from build123d import *

# Parameters (mm, degrees)
SKETCH1_W           = 34
SKETCH1_H           = 103
BOSS_EXTRUDE1_DEPTH = 0.5
SKETCH3_R           = 6.75
SKETCH3_W           = 7
SKETCH3_H           = 3.25
CUT_EXTRUDE1_DEPTH  = 55.242511004


with BuildPart() as part:
    # Sketch1 → Boss-Extrude1 (new, symmetric)
    with BuildSketch(Plane.XY):
        Rectangle(SKETCH1_W, SKETCH1_H)
    extrude(amount=BOSS_EXTRUDE1_DEPTH, both=True)

    # Sketch3 → Cut-Extrude1 (cut, through all)
    with BuildSketch(Plane.XY.offset(0.5)):
        with Locations((-0.255791225, 31.827660642)):
            Circle(SKETCH3_R)
        with Locations((-0.255791225, 10.237617462)):
            Circle(SKETCH3_R)
        with Locations((-0.255791225, -11.352425718)):
            Circle(SKETCH3_R)
        with Locations((-0.25, 45.125)):
            Rectangle(SKETCH3_W, SKETCH3_H)
    extrude(amount=-CUT_EXTRUDE1_DEPTH, mode=Mode.SUBTRACT)


solid = part.part
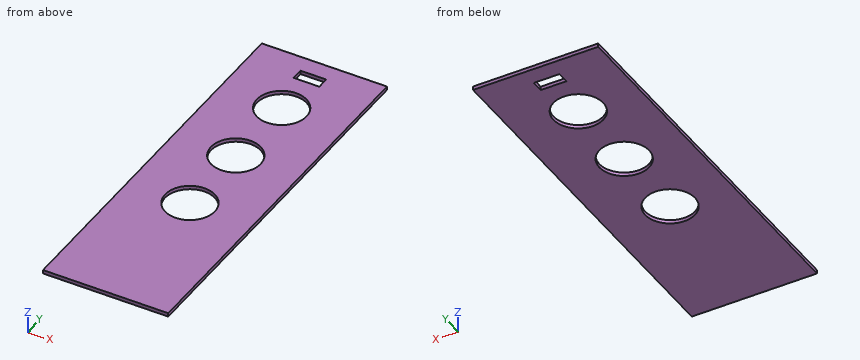
Part model, mm, in its own coordinate system. Round coordinates to 2 decimals unless told otherwise and drop trailing zeros. Write each loop counter-clockwise with the first axis right and the second up, starting at its lowest first coordinate (ties: lowest second). Pieces come first, ordered by that corner, then holes. Notation, with made-up numbers: (75, -20.5) - (108, -20.5) arc R22 cw to (108, 6.5) - close; hole circle Ø2 at (-12.75, 63.25). An arc over 180 degrees is marked (long way). Use CSV: the item, a comma, the result in double quotes.
Item 1: Wall check: L1, parallel to Y at x = 1, z = 0.4; L2, parallel to X at y = 45, z = 0.1; L3, parallel to X at y = -11, z = 0.05 (3 decimals). Give the ranges that are in metal, low to high.
Results list:
L1,"y = -51.5 to -17.98, -4.72 to 3.61, 16.87 to 25.2, 38.46 to 43.5, 46.75 to 51.5"
L2,"x = -17 to -3.75, 3.25 to 17"
L3,"x = -17 to -6.997, 6.485 to 17"
Item 2: Slice it at C-C, the plane y = 33. Write the cut outline in (x, z).
Results list:
outline,"(-17, -0.5) - (-6.9, -0.5) - (-6.9, 0.5) - (-17, 0.5) - close; (6.39, -0.5) - (17, -0.5) - (17, 0.5) - (6.39, 0.5) - close"
Item 3: Flat gauge pin, fed straight in: P1, Ø17.5, axis at x = -0.26, y = -11.35, coming from the -Z side. Where does the tip first touch, or does it go through?
Results list:
P1,"stops at z = -0.5"
Item 4: Slice it at A-A, the plane x = -1. Write the cut outline in (y, z), then the cut area to 3 significant figures.
Results list:
outline,"(-51.5, -0.5) - (-18.06, -0.5) - (-18.06, 0.5) - (-51.5, 0.5) - close; (-4.64, -0.5) - (3.53, -0.5) - (3.53, 0.5) - (-4.64, 0.5) - close; (16.95, -0.5) - (25.12, -0.5) - (25.12, 0.5) - (16.95, 0.5) - close; (38.54, -0.5) - (43.5, -0.5) - (43.5, 0.5) - (38.54, 0.5) - close; (46.75, -0.5) - (51.5, -0.5) - (51.5, 0.5) - (46.75, 0.5) - close"
area,"59.5 mm²"
Item 5: Slice it at D-D, the plane y = -6. Write the cut outline in (x, z), then the cut area to 3 significant figures.
Results list:
outline,"(-17, -0.5) - (-4.37, -0.5) - (-4.37, 0.5) - (-17, 0.5) - close; (3.86, -0.5) - (17, -0.5) - (17, 0.5) - (3.86, 0.5) - close"
area,"25.8 mm²"
Item 6: Slice it at B-B, the plane z = -0.25. Write the cut outline in (x, y), then the cut area to 3 significant figures.
Results list:
outline,"(-17, -51.5) - (17, -51.5) - (17, 51.5) - (-17, 51.5) - close; hole circle Ø13.5 at (-0.26, -11.35); hole circle Ø13.5 at (-0.26, 10.24); hole circle Ø13.5 at (-0.26, 31.83); hole (-3.75, 43.5) - (3.25, 43.5) - (3.25, 46.75) - (-3.75, 46.75) - close"
area,"3,050 mm²"
